Part model, mm, in its own coordinate system. A direction names the side the tool comes from. Give positions to 0.01 mm unless a question says otherwise; leave off trailing zeros. Order: outer loops, then holes, each group sorted by start corner. A loop starts at its lowest first (then second) coordinate and runs counter-clockwise, first axis right, second up. Notation, with made-up numbers: M 20.5,22 L 39.5,22 A9 cw 39.5,33 Z; hole C 35.5,-2.5 d9. An arc over 180 degrees is marked long. One line per question, with ' | ' between items.
```python
from build123d import *

# Parameters (mm, degrees)
SKETCH_R        = 32.393895
PAD_DEPTH       = 12
FILLET_R        = 2
PAD001_DEPTH    = 15
FILLET001_R     = 2
POCKET_DEPTH    = 13
SKETCH003_R     = 7.198044
POCKET001_DEPTH = 13
FILLET002_R     = 1


with BuildPart() as part:
    # Sketch → Pad (new body)
    with BuildSketch(Plane.XY):
        Circle(SKETCH_R)
    extrude(amount=PAD_DEPTH)

    # Fillet
    fillet_edges = [part.edges().sort_by_distance(p)[0] for p in [
        (-32.393895, 0, 12),
    ]]
    fillet(fillet_edges, radius=FILLET_R)

    # Sketch001 (on Face4 of Fillet) → Pad001 (join)
    with BuildSketch(Plane.XY.offset(12)):
        with BuildLine():
            ThreePointArc((7.268672, 23.598905), (0, 27.795475), (-7.268672, 23.598905))
            Line((-7.268672, 23.598905), (-24.071587, -5.504598))
            ThreePointArc((-24.071587, -5.504598), (-24.071587, -13.897737), (-16.802915, -18.094307))
            Line((-16.802915, -18.094307), (16.802915, -18.094307))
            ThreePointArc((16.802915, -18.094307), (24.071587, -13.897737), (24.071587, -5.504598))
            Line((24.071587, -5.504598), (7.268672, 23.598905))
        make_face()
    extrude(amount=PAD001_DEPTH)

    # Fillet001
    fillet001_edges = [part.edges().sort_by_distance(p)[0] for p in [
        (-30.393895, 0, 12),
        (0, 27.795475, 12),
        (-15.67013, 9.047154, 12),
        (-24.071587, -13.897737, 12),
        (0, -18.094307, 12),
        (24.071587, -13.897737, 12),
        (15.67013, 9.047154, 12),
    ]]
    fillet(fillet001_edges, radius=FILLET001_R)

    # Sketch004 (on Face4 of Fillet) → Pocket (cut)
    with BuildSketch(Plane.XY.offset(27)):
        with BuildLine():
            Line((16.879342, 2.224883), (10.371309, 13.497127))
            ThreePointArc((10.371309, 13.497127), (8.97108, 14.2567), (7.659291, 13.352929))
            ThreePointArc((-7.659291, 13.352929), (0, 8.370647), (7.659291, 13.352929))
            ThreePointArc((-7.659291, 13.352929), (-8.97108, 14.2567), (-10.371309, 13.497127))
            Line((-10.371309, 13.497127), (-16.879342, 2.224883))
            ThreePointArc((-16.879342, 2.224883), (-16.837038, 0.632462), (-15.398454, -0.051695))
            ThreePointArc((-7.739163, -13.317976), (-7.254026, -4.193694), (-15.398454, -0.051695))
            ThreePointArc((-7.739163, -13.317976), (-7.865958, -14.905904), (-6.508033, -15.738752))
            Line((-6.508033, -15.738752), (6.508033, -15.738752))
            ThreePointArc((6.508033, -15.738752), (7.865958, -14.905904), (7.739163, -13.317976))
            ThreePointArc((15.398454, -0.051695), (7.254026, -4.193694), (7.739163, -13.317976))
            ThreePointArc((15.398454, -0.051695), (16.837038, 0.632462), (16.879342, 2.224883))
        make_face()
    extrude(amount=-POCKET_DEPTH, mode=Mode.SUBTRACT)

    # Sketch003 (on Face4 of Fillet) → Pocket001 (cut)
    with BuildSketch(Plane.XY.offset(27)):
        with Locations((-15.53568, -8.969529)):
            Circle(SKETCH003_R)
        with Locations((0, 17.939058)):
            Circle(SKETCH003_R)
        with Locations((15.53568, -8.969529)):
            Circle(SKETCH003_R)
    extrude(amount=-POCKET001_DEPTH, mode=Mode.SUBTRACT)

    # Fillet002
    fillet002_edges = [part.edges().sort_by_distance(p)[0] for p in [
        (16.837038, 0.632462, 14),
        (13.625326, 7.861005, 14),
        (8.97108, 14.2567, 14),
        (0, 8.370647, 14),
        (-8.97108, 14.2567, 14),
        (-13.625326, 7.861005, 14),
        (-16.837038, 0.632462, 14),
        (-7.254026, -4.193694, 14),
        (-7.865958, -14.905904, 14),
        (0, -15.738752, 14),
        (7.865958, -14.905904, 14),
        (7.254026, -4.193694, 14),
    ]]
    fillet(fillet002_edges, radius=FILLET002_R)


solid = part.part
```
1. Slice it at A-A on x = 0. Give the cut face in (y, z).
Worked out:
outline: M -32.39,0 L 32.39,0 L 32.39,10 A2 ccw 30.39,12 L 29.8,12 A2 cw 27.8,14 L 27.8,27 L 25.14,27 L 25.14,14 L 10.74,14 L 10.74,27 L 8.37,27 L 8.37,15 A1 cw 7.37,14 L -14.74,14 A1 cw -15.74,15 L -15.74,27 L -18.09,27 L -18.09,14 A2 cw -20.09,12 L -30.39,12 A2 ccw -32.39,10 Z
2. Tool access for faces 4 (the cylindrical face through (16.073, 9.552, 12.57)), 5 (the cylindrical face through (-24.132, -13.791, 20.409)), 6 (the flat face through (0, -18.094, 20)), 7 (the cylindrical face through (24.01, -14, 20.41)), 8 (the flat face through (-16, -9, 14)): list every direction of +Z, -Z, +X, -X, +Y, -Y with a clear straight run to the whole face (end or side of a thin tool).
Worked out:
face 4: +Z, +X, +Y | face 5: +Z, -X | face 6: +Z, +X, -X, -Y | face 7: +Z, +X | face 8: +Z
3. Probe L1, parallel to Y at x = 0, z = 17.5; L2, parallel to Y at x = 3.5, z = 19.75; L3, parallel to X at y = 9, z = 24.25. List the from-to ranges inside material, lowest first. Write a range as from..to.
Worked out:
L1: y = -18.09..-15.74, 8.37..10.74, 25.14..27.8 | L2: y = -18.09..-15.74, 9.14..11.65, 24.23..27.03 | L3: x = -15.7..-12.97, -3.19..3.19, 12.97..15.7
4. Slice it at B-B on z = 21. Give the cut face in (x, y).
Worked out:
outline: M -24.07,-5.5 A8.39 ccw -16.8,-18.09 L 16.8,-18.09 A8.39 ccw 24.07,-5.5 L 7.27,23.6 A8.39 ccw -7.27,23.6 Z; hole C -15.54,-8.97 d14.4; hole M -16.88,2.22 A1.52 ccw -15.4,-0.05 A8.38 cw -7.74,-13.32 A1.52 ccw -6.51,-15.74 L 6.51,-15.74 A1.52 ccw 7.74,-13.32 A8.38 cw 15.4,-0.05 A1.52 ccw 16.88,2.22 L 10.37,13.5 A1.52 ccw 7.66,13.35 A8.38 cw -7.66,13.35 A1.52 ccw -10.37,13.5 Z; hole C 0,17.94 d14.4; hole C 15.54,-8.97 d14.4
5. Slice it at C-C on z = 3.5. Give the cut face in (x, y), then the cut area to 3 significant figures.
Worked out:
outline: C 0,0 d64.79 | area: 3,300 mm2
6. Drop flat-ended pins along their axis: pin 1 (4 mm diameter, centred on x = -4.5, z = 22, fed in from -Y); pin 2 (4 mm diameter, centred on y = 19.5, z = 18.5, fed in from +X); pin 3 (18 mm diameter, centred on x = -13.5, y = 7, fed in from +Z); pin 4 (10 mm diameter, centred on y = 10, z = 3, fed in from +X). Give the stop position or say it passes through.
Worked out:
pin 1: stops at y = -18.09 | pin 2: stops at x = 10.79 | pin 3: stops at z = 27 | pin 4: stops at x = 32.01
7. Mould opens along Y. For faces 1 (the cylindrical face through (-16.85, 0.65, 21.08)), 2 (the cylindrical face through (-16.3, 9.1, 12.6)), 3 (the flat face through (0, 0, 0)) say: released by +Y, released by -Y, zero draft, split by the parting line, or undercut.
Worked out:
face 1: undercut | face 2: released by +Y | face 3: zero draft
